The listing builds one solid part. Answer for the finished solid, in the listing's coordinates (mm). A direction names the side the tool comes from. Give positions to 0.01 mm unless a question says otherwise; leave off trailing zeros. Write each loop counter-clockwise with the first axis right and the second up, starting at its lowest first coordinate (ties: lowest second). Pieces come first, ordered by that corner, then holes.
```python
from build123d import *

# Parameters (mm, degrees)
F0_W     = 20
F0_H     = 10
F1_DEPTH = 20
F3_R     = 2
F4_DEPTH = 5
F5_DEPTH = 5
F2_W     = 3
F2_H     = 5
F6_DEPTH = 49
F2_H_2   = 3
F7_DEPTH = 20
F8_DEPTH = 20


# Not quite as in the source:
# - an extrude ends at something that could not be found from the text; its depth is read off the source's solid


with BuildPart() as f1:
    # F0 (on Top) → F1 (new body)
    with BuildSketch(Plane.XY):
        with Locations((10, 5)):
            Rectangle(F0_W, F0_H)
    extrude(amount=F1_DEPTH)

    # F3 (on face) → F4 (join)
    with BuildSketch(Plane(origin=(0, 0, 0), x_dir=(1, 0, 0), z_dir=(0, 0, -1))):
        with Locations((10, -5)):
            Circle(F3_R)
    extrude(amount=F4_DEPTH)

    # F3 (on face) → F5 (join)
    with BuildSketch(Plane(origin=(0, 0, 0), x_dir=(1, 0, 0), z_dir=(0, 0, -1))):
        with Locations((10, -5)):
            Circle(F3_R)
    extrude(amount=F5_DEPTH)

    # F2 (on face) → F6 (cut, through all)
    with BuildSketch(Plane.XY.offset(20)):
        with Locations((1.5, 5)):
            Rectangle(F2_W, F2_H)
    extrude(amount=-F6_DEPTH, mode=Mode.SUBTRACT)

    # F2 (on face) → F7 (join, through all)
    with BuildSketch(Plane.XY.offset(20)):
        with Locations((1.5, 5)):
            Rectangle(F2_W, F2_H)
        with Locations((10.5, -1.5)):
            Rectangle(F2_W, F2_H_2)
    extrude(amount=-F7_DEPTH)

    # F2 (on face) → F8 (cut, through all)
    with BuildSketch(Plane.XY.offset(20)):
        with Locations((1.5, 5)):
            Rectangle(F2_W, F2_H)
    extrude(amount=-F8_DEPTH, mode=Mode.SUBTRACT)


solid = f1.part
```
Item 1: Consider probe 1 along Y at (x, z) = (1, 14.5); probe 2 along Z at (x, y) = (16, 6.5); probe 3 along Y at (x, z) = (15, 3.75). Determine where each line is inside the solid, lowest interval first.
Conclusion:
probe 1: y = 0 to 2.5, 7.5 to 10
probe 2: z = 0 to 20
probe 3: y = 0 to 10
Item 2: Which of the six approach directions +Z, -Z, +X, -X, +Y, -Y give full straight-line access (tool end or side, diameter ignored) to faces 1 (the face through (16, 0, 10)), 2 (the face through (8.4, 6.2, -2.5)), 3 (the face through (9, -2, 10)), 4 (the face through (1, 2.5, 10))?
Conclusion:
face 1: +Z, -Z, +X, -Y
face 2: -Z
face 3: +Z, -Z, -X, -Y
face 4: +Z, -Z, -X
Item 3: A cutting plane is placed at B-B, the plane x = 10. Give the vertices of the cut face in (y, z).
Conclusion:
outline: (-3, 0) - (3, 0) - (3, -5) - (7, -5) - (7, 0) - (10, 0) - (10, 20) - (-3, 20) - close
Item 4: Each of these flat-tipped pins is pushed along its axis until it touches: P1, Ø0.9, axis at y = -1, z = 11.5, coming from the +X side; P2, Ø2.5, axis at x = 16.5, z = 5, coming from the -Y side; P3, Ø3, axis at x = 9, y = 1, coming from the -Z side. Where does it stop, or does it pass through?
Conclusion:
P1: stops at x = 12
P2: stops at y = 0
P3: stops at z = 0
Item 5: A cutting plane is placed at C-C, the plane z = 8.5. Give the vertices of the cut face in (x, y).
Conclusion:
outline: (0, 0) - (9, 0) - (9, -3) - (12, -3) - (12, 0) - (20, 0) - (20, 10) - (0, 10) - (0, 7.5) - (3, 7.5) - (3, 2.5) - (0, 2.5) - close
Item 6: A cutting plane is placed at A-A, the plane x = 2. Give the vertices of the cut face in (y, z), plus the area to 3 significant figures.
Conclusion:
outline: (0, 0) - (2.5, 0) - (2.5, 20) - (0, 20) - close; (7.5, 0) - (10, 0) - (10, 20) - (7.5, 20) - close
area: 100 mm2
Item 7: Determine the mould class of faces 5 (the face through (4, 0, 10)), 6 (the face through (3, 5, 10)), 7 (the face through (10, 10, 10)) for opening direction Y: pulls with the +Y half, pulls with the -Y half, needs draft (parallel to the pull), parting line crosses it, or undercut.
Conclusion:
face 5: pulls with the -Y half
face 6: undercut
face 7: pulls with the +Y half
Item 8: A cutting plane is placed at D-D, the plane y = 5. Give the vertices of the cut face in (x, z).
Conclusion:
outline: (3, 0) - (8, 0) - (8, -5) - (12, -5) - (12, 0) - (20, 0) - (20, 20) - (3, 20) - close
